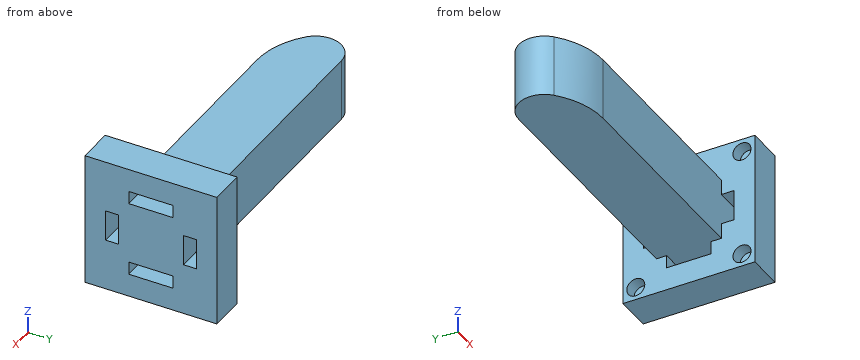
Autodesk Inventor part; units mm, degrees
ref_plane "YZ Plane" through (0, 0, 0) normal (1, 0, 0) x (0, 1, 0)
ref_plane "XZ Plane" through (0, 0, 0) normal (0, 1, 0) x (-1, 0, 0)
ref_plane "XY Plane" through (0, 0, 0) normal (0, 0, 1) x (1, 0, 0)
sketch "Sketch5" plane through (0, 0, 0) normal (0, 0, 1) x (1, 0, 0)
  line L0 (48.5, 0) -> (3.8, 0)
  line L1 (48.5, -12.6) -> (3.8, -12.6)
  line L2 (3.8, -12.6) -> (0, -12.6)
  line L3 (0, -12.6) -> (0, 0)
  line L4 (0, 0) -> (7.8, 0)
  line L5 (38.5, 0) -> (38.5, -12.6)
  line L6 (37.5, -12.6) -> (37.5, 0)
  line L7 (0, -45.1294) -> (0, -34.3361)
  line L8 (0, -34.3361) -> (38.5, -34.3361)
  line L9 (38.5, -34.3361) -> (38.5, -45.1294)
  line L10 (38.5, -45.1294) -> (0, -45.1294)
  line L11 (38.5, -42.4105) -> (39.5, -42.4105)
  line L12 (39.5, -42.4105) -> (39.5, -38.1261)
  line L13 (39.5, -38.1261) -> (38.5, -38.1261)
  line L14 (39.5, -42.4105) -> (39.5, -49.5786)
  line L15 (39.5, -49.5786) -> (45, -49.5786)
  line L16 (45, -49.5786) -> (45, -34.3361)
  line L17 (45, -34.3361) -> (39.5, -34.3361)
  line L18 (39.5, -34.3361) -> (39.5, -38.1261)
  line L19 (48.5, 0) -> (55.8897, 0)
  line L20 (55.8897, 0) -> (55.8897, -12.6)
  line L21 (55.8897, -12.6) -> (48.5, -12.6)
  point P0 (7.8, 0)
  point P1 (39, -42.4105)
  dimension "d63" = 44.7
  dimension "d71" = 0
  dimension "d97" = 12.6
  dimension "d123" = 1
  dimension "d124" = 37.5
  dimension "d125" = 38.5
  dimension "d127" = 1
  dimension "d128" = 5.5
extrude "Extrusion2" add sketch "Sketch5" along normal blind 12 contours L19 L20 L21 L1 L5 L0 | L5 L1 L6 L0 | L6 L1 L2 L3 L4 L0
fillet "Fillet2" radius 15 1 edges at (0, -12.6, 6)
fillet "Rundung3" radius 5 1 edges at (0, 0, 6)
sketch "Skizze17" plane through (55.8897, -12.6, 0) normal (1, 0, 0) x (0, 0, -1)
  line L0 (-19, -6.5) -> (7, -6.5)
  line L1 (7, -6.5) -> (7, 19.1)
  line L2 (7, 19.1) -> (-19, 19.1)
  line L3 (-19, 19.1) -> (-19, -6.5)
  line L4 (-19, -6.5) -> (7, 19.1) construction
  line L5 (7, -6.5) -> (-19, 19.1) construction
  line L6 (0, 12.6) -> (-12, 12.6)
  line L7 (0, 0) -> (-12, 0)
  line L8 (0, 0) -> (0, 12.6)
  line L9 (-12, 0) -> (-12, 12.6)
  point P0 (-6, 6.3)
  point P1 (7, 6.3)
  dimension "d151" = 26
  dimension "d152" = 25.6
  dimension "d153" = 6.5
  dimension "d154" = 6.5
  dimension "d155" = 7
  dimension "d156" = 7
extrude "Extrusion12" add sketch "Skizze17" along normal blind 7 contours L3 L2 L1 L0 | L8 L7 L9 L6
sketch "Skizze18" plane through (55.8897, -12.6, 0) normal (-1, 0, 0) x (0, 0, 1)
  circle A0 centre (-4.5, 16.6) radius 1.75
  circle A1 centre (16.5, 16.6) radius 1.75
  circle A2 centre (16.5, -4) radius 1.75
  circle A3 centre (-4.5, -4) radius 1.75
  line L0 (-7, 19.1) -> (19, 19.1)
  line L1 (-7, -6.5) -> (-7, 19.1)
  line L2 (19, 19.1) -> (19, -6.5)
  line L3 (19, -6.5) -> (-7, -6.5)
  point P0 (0, 12.6)
  dimension "d135" = 3.5
  dimension "d136" = 2.5
  dimension "d137" = 2.5
  dimension "d138" = 3.5
  dimension "d139" = 2.5
  dimension "d140" = 2.5
  dimension "d141" = 2.5
  dimension "d142" = 2.5
  dimension "d143" = 2.5
  dimension "d144" = 2.5
  dimension "d145" = 3.5
  dimension "d146" = 3.5
extrude "Extrusion13" cut sketch "Skizze18" against normal blind 2.5 contours A0 | A1 | A2 | A3
sketch "Skizze22" plane through (55.8897, -12.6, 0) normal (-1, 0, 0) x (0, 0, 1)
  line L0 (0, 12.6) -> (10, 12.6)
  line L1 (9, 15.1) -> (3, 15.1)
  line L2 (-2.5, 10.6) -> (-2.5, 2)
  line L3 (4.6106, -2.5) -> (9, -2.5)
  line L4 (10, -0.0226) -> (9.9863, -0.0226)
  line L5 (9.9863, 12.8711) -> (10, 12.8711)
  line L6 (14.5, 10.6) -> (14.5, 2)
  line L7 (4.6106, -2.5) -> (3, -2.5)
  line L8 (12, 12.6) -> (0, 12.6)
  line L9 (0, 0) -> (0, 12.6)
  line L10 (0, 0) -> (0, 12.6)
  line L11 (0, 12.6) -> (12, 12.6)
  line L12 (0, 0) -> (12, 0)
  line L13 (0, 0) -> (10, 0)
  line L14 (11.3365, 15.1) -> (11.4, 15.1)
  line L15 (3, 15.1) -> (3, 12.6)
  line L16 (0, 10.6) -> (-2.5, 10.6)
  line L17 (10, 10.6) -> (14.5, 10.6)
  line L18 (9, 12.6) -> (9, 15.1)
  line L19 (0, 2) -> (-2.5, 2)
  line L20 (3, 0) -> (3, -2.5)
  line L21 (9, 0) -> (9, -2.5)
  line L22 (10, 2) -> (14.5, 2)
  line L23 (12, 12.6) -> (12, 3.9)
  line L24 (12, 3.9) -> (12, 0)
  line L25 (12, 10.6) -> (12, 1.95)
  line L26 (14.5, 2) -> (14.5, 10.6)
  point P0 (9, 13.85)
  point P1 (3, 13.85)
  point P2 (12.25, 2)
  point P3 (12.25, 10.6)
  point P4 (-1.25, 10.6)
  point P5 (-1.25, 2)
  point P6 (3, 0)
  point P7 (0, 2)
  point P8 (3, 12.6)
  point P9 (9, 12.6)
  point P10 (14.5, 6.3)
  point P11 (12, 2)
  dimension "d172" = 0
  dimension "d173" = 2.5
  dimension "d175" = 2.5
  dimension "d176" = 2.5
  dimension "d180" = 3
  dimension "d181" = 3
  dimension "d183" = 2
  dimension "d184" = 2
  dimension "d185" = 2
  dimension "d186" = 2
  dimension "d190" = 2.5
  dimension "d191" = 3
  dimension "d192" = 3
extrude "Extrusion19" cut sketch "Skizze22" against normal blind 10 contours L15 L1 L18 L0 | L9 L19 L2 L16 | L12 L21 L3 L7 L20 | L17 L6 L22 L24 L23
equation "\"l1\" = 8"
properties part number "Maria_Greifer_3D-Druck"
Verification items for the finished model (mm, model axes). Round coordinates to 2 decimals unless told otherwise and drop trailing zeros. Write each loop counter-clockwise with the first axis right and the second up, starting at its lowest first coordinate (ties: lowest second). Pieces come first, ordered by that corner, then holes. Notation, with made-up numbers: (31, 33) -> (68, 33) arc R20 ccw to (68, 37) -> close; hole circle Ø9 at (79, 58.5). An arc over 180 degrees is marked (long way). Write each question's results on one line, items separated by ' | '.
Q1. Go/stop test with flat-tipped pins: pin 1 Ø1 at (y, z) = (-17, -5) entering from -X; pin 2 Ø3 at (y, z) = (-16.5, 17) entering from -X; pin 3 Ø10 at (x, y) = (34.5, -7) entering from +Z. Record where each tip stops, or that it passes through.
Derived:
pin 1: stops at x = 58.39 | pin 2: stops at x = 55.89 | pin 3: stops at z = 12
Q2. Sectioned sample at B-B, the plane y = -16.6. Record the boundary of the cut face in (x, z).
Derived:
outline: (55.89, -7) -> (62.89, -7) -> (62.89, 19) -> (55.89, 19) -> (55.89, 18.25) -> (58.39, 18.25) -> (58.39, 14.75) -> (55.89, 14.75) -> (55.89, -2.75) -> (58.39, -2.75) -> (58.39, -6.25) -> (55.89, -6.25) -> close
Q3. Sectioned sample at D-D, the plane x = 40.5. Record the boundary of the cut face in (y, z), and give its area (3 significant figures).
Derived:
outline: (-12.6, 0) -> (0, 0) -> (0, 12) -> (-12.6, 12) -> close | area: 151 mm²
Q4. Sectioned sample at A-A, the plane z = 3.75. Record the boundary of the cut face in (x, y).
Derived:
outline: (4.72, -8.7) arc R15 ccw to (14.81, -12.6) -> (62.89, -12.6) -> (62.89, 0) -> (8.08, 0) arc R5 ccw to start; (55.89, -19.1) -> (62.89, -19.1) -> (62.89, -15.1) -> (55.89, -15.1) -> close; (55.89, 2.5) -> (62.89, 2.5) -> (62.89, 6.5) -> (55.89, 6.5) -> close
Q5. Sectioned sample at C-C, the plane z = 11.25. Record the boundary of the cut face in (x, y), and give its area (3 significant figures).
Derived:
outline: (4.72, -8.7) arc R15 ccw to (14.81, -12.6) -> (55.89, -12.6) -> (55.89, -19.1) -> (62.89, -19.1) -> (62.89, 6.5) -> (55.89, 6.5) -> (55.89, 0) -> (8.08, 0) arc R5 ccw to start | area: 819 mm²
Q6. Thickness scan on probe 1 along Y at (x, z) = (56.55, -4.5); probe 2 along Y at (x, z) = (57.5, 6); probe 3 along X at (y, z) = (-9, 16). Record the ranges inside material, lowest first.
Derived:
probe 1: y = -19.1 to -18.35, -14.85 to 2.25, 5.75 to 6.5 | probe 2: y = -19.1 to -15.1, -12.6 to 0, 2.5 to 6.5 | probe 3: x = 55.89 to 62.89
